```python
from build123d import *

# Parameters (mm, degrees)
SKETCH1_R           = 38.1
BOSS_EXTRUDE1_DEPTH = 6.35
FILLET1_R           = 2.54
CUT_EXTRUDE1_START  = -2.54
CUT_EXTRUDE1_DEPTH  = 6.35
SKETCH3_W           = 34.29
SKETCH3_H           = 1.27
SKETCH3_R           = 1.5875
FILLET2_R           = 1.27
SKETCH4_R           = 1.25
CUT_EXTRUDE2_DEPTH  = 6.35
CHAMFER1_SIZE       = 1.27


with BuildPart() as part:
    # Sketch1 → Boss-Extrude1 (new body)
    with BuildSketch(Plane.XY):
        Circle(SKETCH1_R)
        with BuildLine():
            Line((0, 3.753578648), (0, 31.356419273))
            ThreePointArc((0, 31.356419273), (-5.528532606, 30.86519653), (-10.883847669, 29.406919076))
            Line((-10.883847669, 29.406919076), (-7.631535777, 20.619542081))
            Line((-7.631535777, 20.619542081), (-13.336198426, 15.806394174))
            Line((-13.336198426, 15.806394174), (0, 3.753578648))
        make_face(mode=Mode.SUBTRACT)
        with BuildLine():
            Line((20.025215132, 24.12914811), (14.041279368, 16.918874893))
            Line((14.041279368, 16.918874893), (7.020639684, 19.452683713))
            Line((7.020639684, 19.452683713), (3.250694465, 1.876789324))
            Line((3.250694465, 1.876789324), (27.155455662, 15.678209636))
            ThreePointArc((27.155455662, 15.678209636), (23.965777985, 20.220447947), (20.025215132, 24.12914811))
        make_face(mode=Mode.SUBTRACT)
        with BuildLine():
            Line((20.35683811, 3.646289539), (3.250694465, -1.876789324))
            Line((3.250694465, -1.876789324), (27.155455662, -15.678209636))
            ThreePointArc((27.155455662, -15.678209636), (29.494310591, -10.644748583), (30.909062801, -5.277770966))
            Line((30.909062801, -5.277770966), (21.672815145, -3.700667188))
            Line((21.672815145, -3.700667188), (20.35683811, 3.646289539))
        make_face(mode=Mode.SUBTRACT)
        with BuildLine():
            Line((13.336198426, -15.806394174), (0, -3.753578648))
            Line((0, -3.753578648), (0, -31.356419273))
            ThreePointArc((0, -31.356419273), (5.528532606, -30.86519653), (10.883847669, -29.406919076))
            Line((10.883847669, -29.406919076), (7.631535777, -20.619542081))
            Line((7.631535777, -20.619542081), (13.336198426, -15.806394174))
        make_face(mode=Mode.SUBTRACT)
        with BuildLine():
            Line((-7.020639684, -19.452683713), (-3.250694465, -1.876789324))
            Line((-3.250694465, -1.876789324), (-27.155455662, -15.678209636))
            ThreePointArc((-27.155455662, -15.678209636), (-23.965777985, -20.220447947), (-20.025215132, -24.12914811))
            Line((-20.025215132, -24.12914811), (-14.041279368, -16.918874893))
            Line((-14.041279368, -16.918874893), (-7.020639684, -19.452683713))
        make_face(mode=Mode.SUBTRACT)
        with BuildLine():
            Line((-20.35683811, -3.646289539), (-3.250694465, 1.876789324))
            Line((-3.250694465, 1.876789324), (-27.155455662, 15.678209636))
            ThreePointArc((-27.155455662, 15.678209636), (-29.494310591, 10.644748583), (-30.909062801, 5.277770966))
            Line((-30.909062801, 5.277770966), (-21.672815145, 3.700667188))
            Line((-21.672815145, 3.700667188), (-20.35683811, -3.646289539))
        make_face(mode=Mode.SUBTRACT)
    extrude(amount=BOSS_EXTRUDE1_DEPTH)

    # Fillet1
    fillet1_edges = [part.edges().sort_by_distance(p)[0] for p in [
        (0, 3.753578648, 3.175),
        (3.250694465, 1.876789324, 3.175),
        (3.250694465, -1.876789324, 3.175),
        (0, -3.753578648, 3.175),
        (-3.250694465, -1.876789324, 3.175),
        (-3.250694465, 1.876789324, 3.175),
    ]]
    fillet(fillet1_edges, radius=FILLET1_R)

    # Sketch2 → Cut-Extrude1 (cut)
    with BuildSketch(Plane.XY.offset(6.35).offset(CUT_EXTRUDE1_START)):
        with BuildLine():
            Line((-1.956171069, 1.905), (1.956171069, 1.905))
            ThreePointArc((1.956171069, 1.905), (2.7305, 0), (1.956171069, -1.905))
            Line((1.956171069, -1.905), (-1.956171069, -1.905))
            ThreePointArc((-1.956171069, -1.905), (-2.7305, 0), (-1.956171069, 1.905))
        make_face()
    extrude(amount=-CUT_EXTRUDE1_DEPTH, mode=Mode.SUBTRACT)

    # Sketch3 → Cut-Revolve1 (revolve, cut)
    with BuildSketch(Plane(origin=(0, 0, 0), x_dir=(1, 0, 0), z_dir=(0, 1, 0))):
        with Locations((-17.145, -5.715)):
            Rectangle(SKETCH3_W, SKETCH3_H)
        with Locations((-38.1, -3.175)):
            Circle(SKETCH3_R)
    revolve(axis=Axis((0, 0, 1.27), (0, 0, 1)), mode=Mode.SUBTRACT)

    # Fillet2
    fillet2_edges = [part.edges().sort_by_distance(p)[0] for p in [
        (-27.155455662, -15.678209636, 2.54),
        (-7.020639684, -19.452683713, 2.54),
        (-14.041279368, -16.918874893, 2.54),
        (-20.025215132, -24.12914811, 2.54),
        (13.336198426, -15.806394174, 2.54),
        (7.631535777, -20.619542081, 2.54),
        (10.883847669, -29.406919076, 2.54),
        (0, -31.356419273, 2.54),
        (20.35683811, 3.646289539, 2.54),
        (21.672815145, -3.700667188, 2.54),
        (30.909062801, -5.277770966, 2.54),
        (27.155455662, -15.678209636, 2.54),
        (27.155455662, 15.678209636, 2.54),
        (7.020639684, 19.452683713, 2.54),
        (14.041279368, 16.918874893, 2.54),
        (20.025215132, 24.12914811, 2.54),
        (0, 31.356419273, 2.54),
        (-13.336198426, 15.806394174, 2.54),
        (-7.631535777, 20.619542081, 2.54),
        (-10.883847669, 29.406919076, 2.54),
        (-20.35683811, -3.646289539, 2.54),
        (-21.672815145, 3.700667188, 2.54),
        (-30.909062801, 5.277770966, 2.54),
        (-27.155455662, 15.678209636, 2.54),
    ]]
    fillet(fillet2_edges, radius=FILLET2_R)

    # Sketch4 → Cut-Extrude2 (cut)
    with BuildSketch(Plane.XY.offset(5.08)):
        Circle(SKETCH4_R)
    extrude(amount=-CUT_EXTRUDE2_DEPTH, mode=Mode.SUBTRACT)

    # Chamfer1
    chamfer1_edges = [part.edges().sort_by_distance(p)[0] for p in [
        (34.29, 0, 5.08),
    ]]
    chamfer(chamfer1_edges, length=CHAMFER1_SIZE - 0.0001)  # a hair under: the kernel refuses the full size


solid = part.part
```
Source: CAD feature listing. Evaluate the final solid. Frame: model axes, mm. A direction names the side the tool comes from. Round coordinates to 2 decimals unless told otherwise and drop trailing zeros.
(1) Contact query for flat-ended pins moving along their axis: pin 1 Ø4 at (x, y) = (-2, -11.5) entering from +Z; pin 2 Ø12 at (x, y) = (18.5, -7.5) entering from -Z; pin 3 Ø1.5 at (y, z) = (22.5, 1.5) entering from -X; pin 4 Ø1.9 at (x, y) = (-1, 0) entering from -Z. Output: stop coordinate, or through.
From the geometry:
pin 1: stops at z = 5.08
pin 2: stops at z = 0
pin 3: stops at x = -31.28
pin 4: stops at z = 3.81
(2) Access query for faces 1 (the conical face through (-15.3, 29.4, 5.2)), 2 (the cylindrical face through (2.73, 0.03, 1.93)), 3 (the cylindrical face through (-27.008, 15.153, 2.576)). Directions: +Z, -Z, +X, -X, +Y, -Y. A direction counts if a zero-diameter tool reaches every point of the face in a straight line with its end or side. Return the directions, or none.
From the geometry:
face 1: +Z
face 2: -Z
face 3: +Z, -Z
(3) Pull-direction query (X, two-part tool) for faces 4 (the flat face through (16.99, 9.81, 2.5)), 5 (the cylindrical face through (-30.235, -23.183, 0.783)); classes: +X half, -X half, draft (parallel to the pull), parting line (faces both ways), or undercut.
From the geometry:
face 4: undercut
face 5: parting line
(4) Material intervals for probe 1 along X at (y, z) = (20.5, 0.5); probe 2 along Y at (x, z) = (-26.5, 2.25); probe 3 along Y at (x, z) = (-15.5, 4.25), sorted ascending.
From the geometry:
probe 1: x = -32.11 to -7.97, 0 to 17.01, 23.73 to 32.11
probe 2: y = -25.55 to -16.76, -15.5 to 4.52, 15.19 to 25.55
probe 3: y = -33.52 to -18.68, -8.95 to -2.08, 8.95 to 33.52
(5) Section query A-A (y = -13.5). Give the number of separate pieces and of enclosed holes in the cut face, and give its area (3 significant figures).
From the geometry:
separate pieces: 4
enclosed holes: 0
area: 196 mm2
